Read the model definition and answer for the solid it produces. Units are mm, in the model's axes. Face numbers are marked on the shaded views. A direction names the side the tool comes from. Coordinates: 2 decimals unless noted, no trailing zeros. Loops run counter-clockwise (first coordinate to the right, second up) from the corner with the lowest first, then second, coordinate; pieces in that order, holes last. Notation, with made-up numbers: M 52.25,1.5 L 69.25,1.5 A27 cw 69.25,22.5 Z; hole C 75.5,-19 d9. An arc over 180 degrees is marked long. Use one line per item in the form item = value. Start each with the question number.
1. Find the intervals of material crossed by probe 1 along Y at (x, z) = (-4, 13.75); probe 2 along Z at (x, y) = (-27.5, -5.75); probe 3 along Y at (x, z) = (-31.5, 12.5), in increasing order. Write a range as [from, to].
2. The part is cut by section D-D (x = -33). Give the vertices of the cut face in (y, z).
3. For a pull along Y with two mould halves and no side action, classify the marked faces 3, 4 and 5 as released by +Y, released by -Y, zero draft, split by the parting line, or undercut.
4. The part is cut by section C-C (x = -18). Give the vertices of the cut face in (y, z), plus the area to 3 significant figures.
5. Flat-ended cylindrical pins translate along their axes: pin 1 (6 mm diameter, centred on y = -16, z = 12.5, fed in from -X); pin 2 (6 mm diameter, centred on x = -23.5, z = 10, fed in from -Y); pin 3 (10 mm diameter, centred on x = -34, y = -15, fed in from +Z). Find the tip coordinate at first contact, or state that the pin passes through.
6. A tool of negligible diameter and unlimited length cuts with its end or side. For the marked faces 1 and 2, from which of +Z, -Z, +X, -X, +Y, -Y can it reach the whole face along a straight path? Write none if from no direction.
7. The part is cut by section B-B (y = -3.25). Give the vertices of the cut face in (x, z), plus the area to 3 significant figures.
8. The part is cut by section A-A (z = 3.25). Give the vertices of the cut face in (x, y).
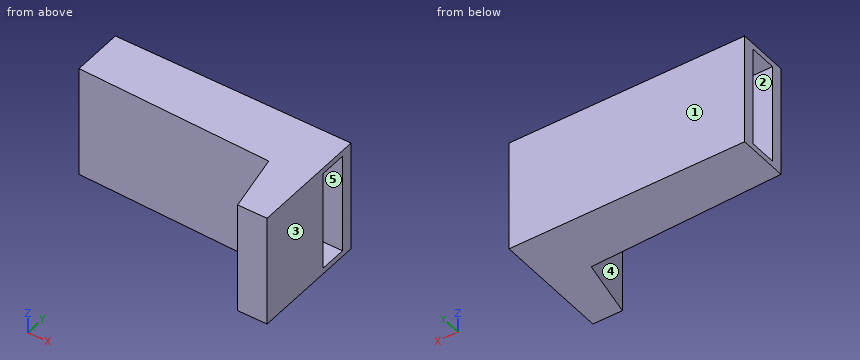
from build123d import *

# Parameters (mm, degrees)
PAD_DEPTH    = 19
SKETCH001_W  = 4.666667
SKETCH001_H  = 17
POCKET_DEPTH = 40.001


with BuildPart() as part:
    # Sketch → Pad (new body)
    with BuildSketch(Plane.XY):
        Polygon((0, 0), (0, -10), (0, -20), (-5, -20), (-7, -9.766667), (-40, -8.666667), (-40, 0), align=None)
    extrude(amount=PAD_DEPTH)

    # Sketch001 → Pocket (cut, through all)
    with BuildSketch(Plane(origin=(-40, 0, 0), x_dir=(0, -1, 0), z_dir=(-1, 0, 0))):
        with Locations((4.333334, 9.5)):
            Rectangle(SKETCH001_W, SKETCH001_H)
    extrude(amount=-POCKET_DEPTH, mode=Mode.SUBTRACT)


solid = part.part
Computed values:
q1.probe_1 = [-20, -6.67], [-2, 0]
q1.probe_2 = [0, 1], [18, 19]
q1.probe_3 = [-8.95, -6.67], [-2, 0]
q2.outline = M -8.9,0 L 0,0 L 0,19 L -8.9,19 Z; hole M -6.67,1 L -2,1 L -2,18 L -6.67,18 Z
q3.face_3 = zero draft
q3.face_4 = released by -Y
q3.face_5 = undercut
q4.outline = M -9.4,0 L 0,0 L 0,19 L -9.4,19 Z; hole M -6.67,1 L -2,1 L -2,18 L -6.67,18 Z
q4.area = 99.3 mm²
q5.pin_1 = -6.37
q5.pin_2 = -9.32
q5.pin_3 = through
q6.face_1 = +Z, -Z, +X, -X, +Y
q6.face_2 = +X, -X
q7.outline = M -40,0 L 0,0 L 0,1 L -40,1 Z; M -40,18 L 0,18 L 0,19 L -40,19 Z
q7.area = 80.0 mm²
q8.outline = M -40,-8.67 L -7,-9.77 L -5,-20 L 0,-20 L 0,-6.67 L -40,-6.67 Z; M -40,-2 L 0,-2 L 0,0 L -40,0 Z
